Geometry check sheet. Reference: the model listing, model coordinates, mm. A direction names the side the tool comes from. Round coordinates to 2 decimals unless told otherwise and drop trailing zeros. Order: outer loops, then holes, each group sorted by start corner. A loop starts at its lowest first (then second) coordinate and runs counter-clockwise, first axis right, second up.
(1) Sectioned sample at C-C (z = 3.5). Record the boundary of the cut face in (x, y), plus the area to 3 significant figures.
(2) Set-up check for faces 1 (the face through (-19.43, 14.4, 1.27)), 2 (the face through (1.5, 12.27, 14.48)): record each of +Z, -Z, +X, -X, +Y, -Y from which the full face is reachable in a straight line by a thin tool's end or side.
(3) Sectioned sample at D-D (z = 13.5). Record the boundary of the cut face in (x, y), plus the area to 3 significant figures.
(4) Release check for a two-part mould opening along X. For faces 3 (the face through (0, 15, 1)), 4 (the face through (20, 7, 1)), 5 (the face through (-2.4, 4.3, 8.1)), 6 (the face through (-20, 7, 1)) record: +X half, -X half, draft (parallel to the pull), parting line (faces both ways), or undercut.
(5) Sectioned sample at A-A (x = -12). Record the boundary of the cut face in (y, z), plus the area to 3 significant figures.
(6) Go/stop test with flat-tipped pins: pin 1 (3 mm diameter, centred on x = -5, z = 8.5, fed in from +Y); pin 2 (2 mm diameter, centred on x = 1.5, y = 7.5, fed in from -Z); pin 3 (7 mm diameter, centred on x = -9.5, y = 11, fed in from +Z); pin 4 (4 mm diameter, centred on x = 4.5, z = 14, fed in from +Y). Record where each tip stops, or that it passes through.
(7) Sectioned sample at B-B (y = 7.5). Give the number of separate pieces and of enclosed holes in the cut face, plus the area to 3 significant figures.
(8) Material ranges on line 1 along X through (y, z) = (7.5, 0.95); line 2 along X through (y, z) = (7.5, 7.25); line 3 along Y through (x, z) = (0, 3.5), recorded low to high.
from build123d import *
from build123d import SkipClean  # not in build123d's __all__

# Parameters (mm, degrees)
F0_W           = 20
F0_H           = 15
F1_DEPTH       = 3
F3_DEPTH       = 10
F5_DEPTH       = 3
F7_DEPTH       = 25
F9_D           = 6
F9_CSINK_D     = 8
F9_CSINK_ANGLE = 90
F10_R          = 2
F12_R          = 0.5


with BuildPart() as f1:
    # F0 (on Top) → F1 (new body)
    with BuildSketch(Plane.XY):
        with Locations((-10, 7.5)):
            Rectangle(F0_W, F0_H)
    extrude(amount=F1_DEPTH)

    # F2 (on face) → F3 (join)
    with BuildSketch(Plane.XY.offset(3)):
        with BuildLine():
            Line((0, 0.5), (0, 14.5))
            ThreePointArc((0, 14.5), (-7, 7.5), (0, 0.5))
        make_face()
    extrude(amount=F3_DEPTH)

    # F4 (on face) → F5 (join)
    with BuildSketch(Plane.XY.offset(13)):
        with BuildLine():
            Line((0, 2.5), (0, 12.5))
            ThreePointArc((0, 12.5), (-5, 7.5), (0, 2.5))
        make_face()
    extrude(amount=F5_DEPTH)

    # F6 (on face) → F7 (cut)
    with BuildSketch(Plane.XY.offset(16)):
        with BuildLine():
            Line((0, 3.5), (0, 11.5))
            ThreePointArc((0, 11.5), (-4, 7.5), (0, 3.5))
        make_face()
    extrude(amount=-F7_DEPTH, mode=Mode.SUBTRACT)

    # F9 (through all)
    with Locations(Plane.XY.offset(3)):
        with Locations((-12, 7.5)):
            CounterSinkHole(F9_D / 2, F9_CSINK_D / 2, counter_sink_angle=F9_CSINK_ANGLE)

    # F10
    f10_edges = [f1.edges().sort_by_distance(p)[0] for p in [
        (-20, 0, 1.5),
        (-20, 15, 1.5),
    ]]
    fillet(f10_edges, radius=F10_R)

    # F11: F1 across plane


with BuildPart() as f1_1:
    add(f1.part, clean=False)
    with SkipClean():  # cleaning this boolean's faces spoils the solid; the shape is the same uncleaned
        add(f1.part.mirror(Plane.YZ), clean=False)

    # F12
    f12_edges = [f1_1.edges().sort_by_distance(p)[0] for p in [
        (-9, 0, 3),
        (9, 0, 3),
    ]]
    fillet(f12_edges, radius=F12_R)


solid = f1_1.part
Answer below:
1. outline: circle Ø14 at (0, 7.5); hole circle Ø8 at (0, 7.5)
1. area: 104 mm2
2. face 1: +Z, -Z, -X, +Y
2. face 2: +Z
3. outline: circle Ø10 at (0, 7.5); hole circle Ø8 at (0, 7.5)
3. area: 28.3 mm2
4. face 3: draft
4. face 4: +X half
4. face 5: undercut
4. face 6: -X half
5. outline: (0, 0) - (4.5, 0) - (4.5, 2) - (3.5, 3) - (0.5, 3) arc R0.5 ccw to (0, 2.5) - close; (10.5, 0) - (15, 0) - (15, 2.5) arc R0.5 ccw to (14.5, 3) - (11.5, 3) - (10.5, 2) - close
5. area: 25.9 mm2
6. pin 1: stops at y = 13.56
6. pin 2: passes through
6. pin 3: stops at z = 13
6. pin 4: stops at y = 13.93
7. separate pieces: 4
7. enclosed holes: 0
7. area: 124 mm2
8. line 1: x = -20 to -15, -9 to -4, 4 to 9, 15 to 20
8. line 2: x = -7 to -4, 4 to 7
8. line 3: y = 0.5 to 3.5, 11.5 to 14.5
